Can you work these out from the model? Positions are in its coordinate system, mm. A direction names the side the tool comes from. Coordinates: 2 decimals unless noted, no trailing zeros. Loops run counter-clockwise (first coordinate to the right, second up) from the corner with the lowest first, then second, coordinate; pieces in that order, holes last. Notation, with made-up numbers: (63.5, 62) -> (105.5, 62) arc R23 cw to (105.5, 73) -> close; hole circle Ø2 at (37.25, 71). An arc over 180 degrees is marked (long way). Use one line per item in the form item = value. Start each with the question number.
(1) I'm going to push flat-ended pins straight in: pin 1 (3.5 mm diameter, centred on x = 15.875, z = 0, fed in from -Y); pin 2 (6 mm diameter, centred on x = -6.223, y = -27.051, fed in from +Z) (3 decimals). Where does each tip first touch, or does it pass through?
(2) On a 3-axis mill with a long thin cutter (end or side, diameter ignored), from which of +Z, -Z, +X, -X, +Y, -Y can I reach the whole of each face in a straight line? I mean faces 5 (the cylindrical face through (-14.064, -25.267, -0.57)), 6 (the flat face through (17.16, 29.99, 0.04)), 7 (the flat face through (5.5, 12.7, 0)). Say none if no direction works.
(3) I need wall thicknesses on line 1 (Y direction, x = -7, z = -2.75) (3 decimals); line 2 (Y direction, x = 5, z = 2.5) (3 decimals); line 3 (X direction, y = -17.5, z = 0.5) (3 decimals). Which ranges of each line are inside material? Lowest first, please. Write a range as [from, to].
(4) Thinking about a two-plate mould opening in Y: for faces 1 (the cylindrical face through (-7.6, -24.9, 0)), 2 (the flat face through (-5.474, 19.094, 0.044)), 3 (the conical face through (15.57, -14.932, 0.126)), 4 (the flat face through (0, 0, 3.175)), which applies, released by +Y, released by -Y, zero draft, split by the parting line, or undercut?
(5) Imagine slicing it at C-C (x = -8). List the corners of the cut face in (y, z) for me (3 decimals).
(6) Imagine slicing it at D-D (y = 31). List the corners of the cut face in (x, z) for me (3 decimals), plus the area to 3 significant figures.
(7) Imagine slicing it at A-A (x = -3). List the corners of the cut face in (y, z) for me (3 decimals).
(8) Imagine slicing it at B-B (y = 20.5). List the corners of the cut face in (x, z) for me (3 decimals).
```python
from build123d import *

# Parameters (mm, degrees)
SKETCH1_W                      = 44.45
SKETCH1_H                      = 69.85
BOSS_EXTRUDE1_DEPTH            = 3.175
CHAMFER1_SIZE                  = 10
CUT_EXTRUDE1_DEPTH             = 7.35
TAP_DRILL_FOR_10_24_TAP1_D     = 3.7973
TAP_DRILL_FOR_10_24_TAP1_DEPTH = 19.05
TAP_DRILL_FOR_10_24_TAP1_TIP   = 1.140824014
F_10_CLEARANCE_HOLE1_D         = 5.1054
F_10_CLEARANCE_HOLE1_DEPTH     = 12.7
F_10_CLEARANCE_HOLE1_TIP       = 1.533816902
FILLET1_R                      = 2.54


with BuildPart() as part:
    # Sketch1 → Boss-Extrude1 (new body, symmetric)
    with BuildSketch(Plane.XY):
        Rectangle(SKETCH1_W, SKETCH1_H)
    extrude(amount=BOSS_EXTRUDE1_DEPTH, both=True)

    # Chamfer1
    chamfer1_edges = [part.edges().sort_by_distance(p)[0] for p in [
        (-22.225, 34.925, 0),
        (22.225, 34.925, 0),
    ]]
    chamfer(chamfer1_edges, length=CHAMFER1_SIZE)

    # Sketch2 → Cut-Extrude1 (cut, through all)
    with BuildSketch(Plane.XY.offset(3.175)):
        Polygon((7.332348419, 15.875), (3.666174209, 22.225), (-3.666174209, 22.225), (-7.332348419, 15.875), (-3.666174209, 9.525), (3.666174209, 9.525), align=None)
    extrude(amount=-CUT_EXTRUDE1_DEPTH, mode=Mode.SUBTRACT)

    # Tap Drill for #10-24 Tap1
    with Locations(Plane(origin=(0, -34.925, 0), x_dir=(-1, 0, 0), z_dir=(0, -1, 0))):
        with Locations((15.875, 0), (-15.875, 0)):
            Hole(TAP_DRILL_FOR_10_24_TAP1_D / 2, depth=TAP_DRILL_FOR_10_24_TAP1_DEPTH)
            with Locations((0, 0, -(TAP_DRILL_FOR_10_24_TAP1_DEPTH + TAP_DRILL_FOR_10_24_TAP1_TIP / 2))):  # 118° drill point
                Cone(0, TAP_DRILL_FOR_10_24_TAP1_D / 2, TAP_DRILL_FOR_10_24_TAP1_TIP, mode=Mode.SUBTRACT)

    # #10 Clearance Hole1
    with Locations(Plane.XY.offset(3.175)):
        with Locations((-6.223, -14.351), (6.223, -14.351), (6.223, -27.051), (-6.223, -27.051)):
            Hole(F_10_CLEARANCE_HOLE1_D / 2, depth=F_10_CLEARANCE_HOLE1_DEPTH)
            with Locations((0, 0, -(F_10_CLEARANCE_HOLE1_DEPTH + F_10_CLEARANCE_HOLE1_TIP / 2))):  # 118° drill point
                Cone(0, F_10_CLEARANCE_HOLE1_D / 2, F_10_CLEARANCE_HOLE1_TIP, mode=Mode.SUBTRACT)

    # Fillet1
    fillet1_edges = [part.edges().sort_by_distance(p)[0] for p in [
        (22.225, -34.925, 0),
        (-22.225, -34.925, 0),
    ]]
    fillet(fillet1_edges, radius=FILLET1_R)


solid = part.part
```
Worked out:
q1.pin_1 = -15.79
q1.pin_2 = 3.175
q2.face_5 = -Y
q2.face_6 = +Z, -Z, +X, +Y
q2.face_7 = +Z, -Z
q3.line_1 = [-34.925, -29.483], [-24.619, -16.783], [-11.919, 15.299], [16.451, 34.925]
q3.line_2 = [-34.925, -29.292], [-24.81, -16.592], [-12.11, 11.835], [19.915, 34.925]
q3.line_3 = [-22.225, -17.707], [-14.043, 14.043], [17.707, 22.225]
q4.face_1 = undercut
q4.face_2 = undercut
q4.face_3 = released by -Y
q4.face_4 = zero draft
q5.outline = (-34.925, -3.175) -> (-28.884, -3.175) -> (-28.884, 3.175) -> (-34.925, 3.175) -> close; (-25.218, -3.175) -> (-16.184, -3.175) -> (-16.184, 3.175) -> (-25.218, 3.175) -> close; (-12.518, -3.175) -> (34.925, -3.175) -> (34.925, 3.175) -> (-12.518, 3.175) -> close
q6.outline = (-16.15, -3.175) -> (16.15, -3.175) -> (16.15, 3.175) -> (-16.15, 3.175) -> close
q6.area = 205 mm2
q7.outline = (-34.925, -3.175) -> (9.525, -3.175) -> (9.525, 3.175) -> (-34.925, 3.175) -> close; (22.225, -3.175) -> (34.925, -3.175) -> (34.925, 3.175) -> (22.225, 3.175) -> close
q8.outline = (-22.225, -3.175) -> (-4.662, -3.175) -> (-4.662, 3.175) -> (-22.225, 3.175) -> close; (4.662, -3.175) -> (22.225, -3.175) -> (22.225, 3.175) -> (4.662, 3.175) -> close
